```python
from build123d import *

# Parameters (mm, degrees)
SKETCH064_R   = 5
SKETCH064_R_2 = 2
PAD034_DEPTH  = 2.5
SKETCH065_W   = 1
SKETCH065_H   = 42
PAD035_DEPTH  = 1.5
SKETCH093_R   = 2.5
SKETCH093_R_2 = 1
PAD058_DEPTH  = 5.5
FILLET001_R   = 1
FILLET002_R   = 1.5
CHAMFER_SIZE  = 1.5


with BuildPart() as part:
    # Sketch064 (on DatumPlane) → Pad034 (new body)
    with BuildSketch(Plane(origin=(1.5, 0.401924, 0), x_dir=(0.866025, 0.5, 0), z_dir=(0.5, -0.866025, 0))):
        with BuildLine():
            Line((56, 26.06023), (56, -26.06023))
            ThreePointArc((51.30847, -30), (54.572341, -29.123408), (56, -26.06023))
            Line((51.30847, -30), (20.677938, -24.623561))
            ThreePointArc((20.677938, 24.623561), (0, 0), (20.677938, -24.623561))
            Line((20.677938, 24.623561), (51.30847, 30))
            ThreePointArc((56, 26.06023), (54.572341, 29.123408), (51.30847, 30))
        make_face()
        with Locations((37, 0)):
            Circle(SKETCH064_R, mode=Mode.SUBTRACT)
        with Locations((52, 26.06023)):
            Circle(SKETCH064_R_2, mode=Mode.SUBTRACT)
        with Locations((52, -26.06023)):
            Circle(SKETCH064_R_2, mode=Mode.SUBTRACT)
        with Locations((14.5, -18.186533)):
            Circle(SKETCH064_R_2, mode=Mode.SUBTRACT)
        with Locations((14.5, 18.186533)):
            Circle(SKETCH064_R_2, mode=Mode.SUBTRACT)
        with BuildLine():
            ThreePointArc((24.501937, 21.226197), (21.091285, 16.363333), (25.954149, 12.952681))
            Line((25.954149, 12.952681), (41.713229, 15.7188))
            ThreePointArc((41.713229, 15.7188), (45.123881, 20.581665), (40.261016, 23.992317))
            Line((40.261016, 23.992317), (24.501937, 21.226197))
        make_face(mode=Mode.SUBTRACT)
        with BuildLine():
            ThreePointArc((25.954149, -12.952681), (21.091285, -16.363333), (24.501937, -21.226197))
            Line((24.501937, -21.226197), (40.261016, -23.992317))
            ThreePointArc((40.261016, -23.992317), (45.123881, -20.581665), (41.713229, -15.7188))
            Line((41.713229, -15.7188), (25.954149, -12.952681))
        make_face(mode=Mode.SUBTRACT)
        with BuildLine():
            ThreePointArc((9.8, -8), (14, -12.2), (18.2, -8))
            Line((18.2, -8), (18.2, 8))
            ThreePointArc((18.2, 8), (14, 12.2), (9.8, 8))
            Line((9.8, 8), (9.8, -8))
        make_face(mode=Mode.SUBTRACT)
    extrude(amount=PAD034_DEPTH)

    # Sketch065 (on DatumPlane) → Pad035 (join)
    with BuildSketch(Plane(origin=(1.5, 0.401924, 0), x_dir=(0.866025, 0.5, 0), z_dir=(0.5, -0.866025, 0))):
        with BuildLine():
            ThreePointArc((9.509118, 16.041278), (2.7, 0), (9.509118, -16.041278))
            Line((10.203777, -15.321938), (9.509118, -16.041278))
            ThreePointArc((10.203777, 15.321938), (3.7, 0), (10.203777, -15.321938))
            Line((9.509118, 16.041278), (10.203777, 15.321938))
        make_face()
        with Locations((52.8, 0)):
            Rectangle(SKETCH065_W, SKETCH065_H)
        Polygon((18.720112, 21.538636), (46.298501, 26.379346), (46.471383, 25.394403), (18.892994, 20.553694), align=None)
        Polygon((18.720112, -21.538636), (46.298501, -26.379346), (46.471383, -25.394403), (18.892994, -20.553694), align=None)
    extrude(amount=-PAD035_DEPTH)

    # Sketch093 (on DatumPlane) → Pad058 (join)
    with BuildSketch(Plane(origin=(1.5, 0.401924, 0), x_dir=(0.866025, 0.5, 0), z_dir=(0.5, -0.866025, 0))):
        with Locations((22, 8)):
            Circle(SKETCH093_R)
        with Locations((22, 8)):
            Circle(SKETCH093_R_2, mode=Mode.SUBTRACT)
        with Locations((47, 12)):
            Circle(SKETCH093_R)
        with Locations((47, 12)):
            Circle(SKETCH093_R_2, mode=Mode.SUBTRACT)
        with Locations((47, -12)):
            Circle(SKETCH093_R)
        with Locations((47, -12)):
            Circle(SKETCH093_R_2, mode=Mode.SUBTRACT)
        with Locations((22, -8)):
            Circle(SKETCH093_R)
        with Locations((22, -8)):
            Circle(SKETCH093_R_2, mode=Mode.SUBTRACT)
    extrude(amount=-PAD058_DEPTH)

    # Fillet001
    fillet001_edges = [part.edges().sort_by_distance(p)[0] for p in [
        (14.874356, 5.23686, 12.2),
        (18.511662, 7.33686, 0),
        (14.874356, 5.23686, -12.2),
        (11.237049, 3.13686, 0),
        (21.015588, 8.782503, -16.363333),
        (32.050834, 15.153705, -14.335741),
        (41.828427, 20.798801, -20.581665),
        (30.793181, 14.427598, -22.609257),
        (32.050834, 15.153705, 14.335741),
        (41.828427, 20.798801, 20.581665),
        (30.793181, 14.427598, 22.609257),
        (21.015588, 8.782503, 16.363333),
    ]]
    fillet(fillet001_edges, radius=FILLET001_R)

    # Fillet002
    fillet002_edges = [part.edges().sort_by_distance(p)[0] for p in [
        (2.75, -1.76314, 0),
    ]]
    fillet(fillet002_edges, radius=FILLET002_R)

    # Chamfer
    chamfer_edges = [part.edges().sort_by_distance(p)[0] for p in [
        (13.575318, 4.48686, -18.186533),
        (13.575318, 4.48686, 18.186533),
        (46.05127, 23.23686, 26.06023),
        (46.05127, 23.23686, -26.06023),
    ]]
    chamfer(chamfer_edges, length=CHAMFER_SIZE)


solid = part.part
```
Input: part model. Units: mm. Frame: model coordinates. A direction names the side the tool comes from. Give positions to 0.01 mm unless a question says otherwise; leave off trailing zeros. Use a Markdown table: item, result.
Q1. First-contact query: P1, Ø8, axis at x = 28.5, y = 13.5, coming from the +Z side; P2, Ø12, axis at x = 44.5, z = 11.5, coming from the -Y side; P3, Ø5, axis at x = 17.5, z = 4, coming from the +Y side. Flat tips, straight axial feed; report the tip coordinate or a pass-through.
Entries:
| item | result |
|---|---|
| P1 | stops at z = 26.92 |
| P2 | stops at y = 18.88 |
| P3 | stops at y = 16.89 |
Q2. Pull-direction query (Z, two-part tool) for faces 1 (the cylindrical face through (48.975, 27.242, -29.155)), 2 (the flat face through (42.2, 23.9, -12)), 3 (the flat face through (9.66, 5.97, 15.69)); classes: pulls with the +Z half, pulls with the -Z half, needs draft (parallel to the pull), parting line crosses it, or undercut.
Entries:
| item | result |
|---|---|
| face 1 | pulls with the -Z half |
| face 2 | undercut |
| face 3 | pulls with the +Z half |
Q3. Access query for faces 4 (the flat face through (46.423, 27.192, -0.294)), 5 (the flat face through (10.357, 4.662, 0.112)), 6 (the cylindrical face through (10.834, 3.233, -0.112)). Directions: +Z, -Z, +X, -X, +Y, -Y. A direction counts if a zero-diameter tool reaches every point of the face in a straight line with its end or side. Return the directions, or none.
Entries:
| item | result |
|---|---|
| face 4 | +Z, -Z |
| face 5 | +X, +Y |
| face 6 | +X |
Q4. Section query A-A, the plane z = 1.5. State how many separate pieces and enclosed holes the cut face has, plus the area to 3 significant figures.
Entries:
| item | result |
|---|---|
| separate pieces | 3 |
| enclosed holes | 0 |
| area | 96.6 mm² |
Q5. Ray query, probe 1 along Z at (x, y) = (46.5, 25); probe 2 along Y at (x, z) = (37, -8); probe 3 along X at (y, z) = (4, 10). Return the intervals inside material, ascending. Write a range as from..to.
Entries:
| item | result |
|---|---|
| probe 1 | z = -29.98..-28.18, -23.99..23.99, 28.18..29.98 |
| probe 2 | y = 18.01..20.9 |
| probe 3 | x = 5.27..6.57, 7.73..11.27 |
